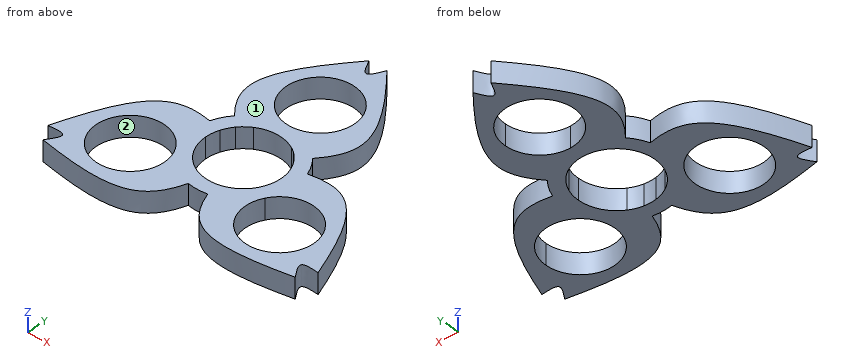
```python
from build123d import *

# Parameters (mm, degrees)
F0_R     = 9.95
F1_DEPTH = 6


with BuildPart() as f1:
    # F0 (on Top) → F1 (new body)
    with BuildSketch(Plane.XY):
        with BuildLine():
            ThreePointArc((5.5, 9.5262794416), (6.3093407999, 9.0106724872), (7.0706637066, 8.4264888743))
            ThreePointArc((7.0706637066, 8.4264888743), (7.8268557987, 7.7291867817), (8.5146077493, 6.9642985918))
            add(Edge.make_bspline(
                [(8.5146077493, 6.9642985918), (9.5301249028, 7.9008868503), (10.4822945034, 8.8485192108), (11.3460669028, 9.8115628642)],
                knots=[0.1806363612, 0.1806363612, 0.1806363612, 0.1806363612, 0.2520657546, 0.2520657546, 0.2520657546, 0.2520657546], degree=3))
            add(Edge.make_bspline(
                [(11.3460669028, 9.8115628642), (13.9736725709, 12.7411528396), (19.7429640918, 22.5358646022), (10.0301146668, 35.0297546933), (2.6054169788, 43.7370347171)],
                knots=[0.2520657546, 0.2520657546, 0.2520657546, 0.2520657546, 0.4693547987, 0.9448204936, 0.9448204936, 0.9448204936, 0.9448204936], degree=3))
            add(Edge.make_bspline(
                [(-2.6054169788, 43.7370347171), (-1.7369446525, 41.8435173586), (0, 38.0564826414), (1.7369446525, 41.8435173586), (2.6054169788, 43.7370347171)],
                knots=[0, 0, 0, 0, 0.5, 1, 1, 1, 1], degree=3))
            add(Edge.make_bspline(
                [(-11.3460669028, 9.8115628642), (-13.9736725709, 12.7411528396), (-19.7429640918, 22.5358646022), (-10.0301146668, 35.0297546933), (-2.6054169788, 43.7370347171)],
                knots=[0.2520657546, 0.2520657546, 0.2520657546, 0.2520657546, 0.4693547987, 0.9448204936, 0.9448204936, 0.9448204936, 0.9448204936], degree=3))
            add(Edge.make_bspline(
                [(-8.5146077493, 6.9642985918), (-9.5301249028, 7.9008868503), (-10.4822945034, 8.8485192108), (-11.3460669028, 9.8115628642)],
                knots=[0.1806363612, 0.1806363612, 0.1806363612, 0.1806363612, 0.2520657546, 0.2520657546, 0.2520657546, 0.2520657546], degree=3))
            ThreePointArc((-8.5146077493, 6.9642985918), (-7.1234292346, 8.381930323), (-5.5, 9.5262794416))
            ThreePointArc((-5.5, 9.5262794416), (0, 11), (5.5, 9.5262794416))
        make_face()
        with BuildLine():
            ThreePointArc((0, 15.05), (-7.0357124728, 32.0357124728), (9.95, 25))
            ThreePointArc((9.95, 25), (7.0357124728, 17.9642875272), (0, 15.05))
        make_face(mode=Mode.SUBTRACT)
        with BuildLine():
            add(Edge.make_bspline(
                [(8.5146077493, 6.9642985918), (9.5301249028, 7.9008868503), (10.4822945034, 8.8485192108), (11.3460669028, 9.8115628642)],
                knots=[0.1806363612, 0.1806363612, 0.1806363612, 0.1806363612, 0.2520657546, 0.2520657546, 0.2520657546, 0.2520657546], degree=3))
            ThreePointArc((8.5146077493, 6.9642985918), (9.5262794416, 5.5), (10.2885633747, 3.8917173182))
            add(Edge.make_bspline(
                [(10.2885633747, 3.8917173182), (11.6074311762, 4.3028868419), (12.9041896741, 4.6536737245), (14.1700961426, 4.9202007387)],
                knots=[0.1806363612, 0.1806363612, 0.1806363612, 0.1806363612, 0.2520657546, 0.2520657546, 0.2520657546, 0.2520657546], degree=3))
            ThreePointArc((14.1700961426, 4.9202007387), (12.9903810568, 7.5), (11.3460669028, 9.8115628642))
        make_face()
        with BuildLine():
            add(Edge.make_bspline(
                [(10.2885633747, 3.8917173182), (11.6074311762, 4.3028868419), (12.9041896741, 4.6536737245), (14.1700961426, 4.9202007387)],
                knots=[0.1806363612, 0.1806363612, 0.1806363612, 0.1806363612, 0.2520657546, 0.2520657546, 0.2520657546, 0.2520657546], degree=3))
            ThreePointArc((10.2885633747, 3.8917173182), (10.8206792098, 1.9781055177), (11, 0))
            ThreePointArc((11, 0), (9.5262794416, -5.5), (5.5, -9.5262794416))
            ThreePointArc((5.5, -9.5262794416), (3.6972499752, -10.3600358407), (1.7739556254, -10.85601591))
            add(Edge.make_bspline(
                [(1.7739556254, -10.85601591), (2.0773062734, -12.2037736923), (2.4218951707, -13.5021929353), (2.8240292398, -14.7317636029)],
                knots=[0.1806363612, 0.1806363612, 0.1806363612, 0.1806363612, 0.2520657546, 0.2520657546, 0.2520657546, 0.2520657546], degree=3))
            add(Edge.make_bspline(
                [(2.8240292398, -14.7317636029), (4.0473257472, -18.4721318504), (9.6451491958, -28.3658407506), (25.3216001194, -26.201211451), (36.5746746618, -24.1248746496)],
                knots=[0.2520657546, 0.2520657546, 0.2520657546, 0.2520657546, 0.4693547987, 0.9448204936, 0.9448204936, 0.9448204936, 0.9448204936], degree=3))
            add(Edge.make_bspline(
                [(36.5746746618, -24.1248746496), (35.3690766899, -22.4259968733), (32.9578807462, -19.0282413207), (37.1060213425, -19.4175204852), (39.1800916406, -19.6121600675)],
                knots=[0, 0, 0, 0, 0.5, 1, 1, 1, 1], degree=3))
            add(Edge.make_bspline(
                [(14.1700961426, 4.9202007387), (18.0209983181, 5.7309790107), (29.3881132876, 5.8299761484), (35.3517147861, -8.8285432423), (39.1800916406, -19.6121600675)],
                knots=[0.2520657546, 0.2520657546, 0.2520657546, 0.2520657546, 0.4693547987, 0.9448204936, 0.9448204936, 0.9448204936, 0.9448204936], degree=3))
        make_face()
        with BuildLine():
            ThreePointArc((13.033682327, -7.525), (24.2258845934, -2.8890380284), (31.6006350946, -12.5))
            ThreePointArc((31.6006350946, -12.5), (19.0753855958, -22.1109619716), (13.033682327, -7.525))
        make_face(mode=Mode.SUBTRACT)
        with BuildLine():
            ThreePointArc((-10.2885633747, 3.8917173182), (-9.5262794416, 5.5), (-8.5146077493, 6.9642985918))
            add(Edge.make_bspline(
                [(-8.5146077493, 6.9642985918), (-9.5301249028, 7.9008868503), (-10.4822945034, 8.8485192108), (-11.3460669028, 9.8115628642)],
                knots=[0.1806363612, 0.1806363612, 0.1806363612, 0.1806363612, 0.2520657546, 0.2520657546, 0.2520657546, 0.2520657546], degree=3))
            ThreePointArc((-11.3460669028, 9.8115628642), (-12.9903810568, 7.5), (-14.1700961426, 4.9202007387))
            add(Edge.make_bspline(
                [(-10.2885633747, 3.8917173182), (-11.6074311762, 4.3028868419), (-12.9041896741, 4.6536737245), (-14.1700961426, 4.9202007387)],
                knots=[0.1806363612, 0.1806363612, 0.1806363612, 0.1806363612, 0.2520657546, 0.2520657546, 0.2520657546, 0.2520657546], degree=3))
        make_face()
        with BuildLine():
            add(Edge.make_bspline(
                [(1.7739556254, -10.85601591), (2.0773062734, -12.2037736923), (2.4218951707, -13.5021929353), (2.8240292398, -14.7317636029)],
                knots=[0.1806363612, 0.1806363612, 0.1806363612, 0.1806363612, 0.2520657546, 0.2520657546, 0.2520657546, 0.2520657546], degree=3))
            ThreePointArc((1.7739556254, -10.85601591), (0, -11), (-1.7739556254, -10.85601591))
            add(Edge.make_bspline(
                [(-1.7739556254, -10.85601591), (-2.0773062734, -12.2037736923), (-2.4218951707, -13.5021929353), (-2.8240292398, -14.7317636029)],
                knots=[0.1806363612, 0.1806363612, 0.1806363612, 0.1806363612, 0.2520657546, 0.2520657546, 0.2520657546, 0.2520657546], degree=3))
            ThreePointArc((-2.8240292398, -14.7317636029), (0, -15), (2.8240292398, -14.7317636029))
        make_face()
        with BuildLine():
            ThreePointArc((-11, 0), (-10.8206792098, 1.9781055177), (-10.2885633747, 3.8917173182))
            add(Edge.make_bspline(
                [(-10.2885633747, 3.8917173182), (-11.6074311762, 4.3028868419), (-12.9041896741, 4.6536737245), (-14.1700961426, 4.9202007387)],
                knots=[0.1806363612, 0.1806363612, 0.1806363612, 0.1806363612, 0.2520657546, 0.2520657546, 0.2520657546, 0.2520657546], degree=3))
            add(Edge.make_bspline(
                [(-14.1700961426, 4.9202007387), (-18.0209983181, 5.7309790107), (-29.3881132876, 5.8299761484), (-35.3517147861, -8.8285432423), (-39.1800916406, -19.6121600675)],
                knots=[0.2520657546, 0.2520657546, 0.2520657546, 0.2520657546, 0.4693547987, 0.9448204936, 0.9448204936, 0.9448204936, 0.9448204936], degree=3))
            add(Edge.make_bspline(
                [(-39.1800916406, -19.6121600675), (-37.1060213425, -19.4175204852), (-32.9578807462, -19.0282413207), (-35.3690766899, -22.4259968733), (-36.5746746618, -24.1248746496)],
                knots=[0, 0, 0, 0, 0.5, 1, 1, 1, 1], degree=3))
            add(Edge.make_bspline(
                [(-2.8240292398, -14.7317636029), (-4.0473257472, -18.4721318504), (-9.6451491958, -28.3658407506), (-25.3216001194, -26.201211451), (-36.5746746618, -24.1248746496)],
                knots=[0.2520657546, 0.2520657546, 0.2520657546, 0.2520657546, 0.4693547987, 0.9448204936, 0.9448204936, 0.9448204936, 0.9448204936], degree=3))
            add(Edge.make_bspline(
                [(-1.7739556254, -10.85601591), (-2.0773062734, -12.2037736923), (-2.4218951707, -13.5021929353), (-2.8240292398, -14.7317636029)],
                knots=[0.1806363612, 0.1806363612, 0.1806363612, 0.1806363612, 0.2520657546, 0.2520657546, 0.2520657546, 0.2520657546], degree=3))
            ThreePointArc((-1.7739556254, -10.85601591), (-3.6972499752, -10.3600358407), (-5.5, -9.5262794416))
            ThreePointArc((-5.5, -9.5262794416), (-9.5262794416, -5.5), (-11, 0))
        make_face()
        with Locations((-21.6506350946, -12.5)):
            Circle(F0_R, mode=Mode.SUBTRACT)
    extrude(amount=F1_DEPTH)


solid = f1.part
```
Geometry check sheet. Reference: the model listing, model coordinates, mm. Face numbers are marked on the shaded views. Coordinates: 2 decimals unless noted, no trailing zeros. Answer in a Markdown table with one row per item. Add a question column.
1. Gauge pin test, flat ends, axial feed: pin 1 Ø2 at (x, z) = (28, 1) entering from +Y; pin 2 Ø1 at (y, z) = (-12.5, 4) entering from -X; pin 3 Ø2 at (y, z) = (11, 3.5) entering from -X. Record the tip position at first contact, or that the pin passes through.
2. Draft check along Y on the marked faces 1 and 2. Enter one of: +Y half, -Y half, draft (parallel to the pull), parting line (faces both ways), or undercut.
3. Section check A-A (x = -13). Give the number of separate pieces and of enclosed holes in the cut face, plus the area to 3 significant figures.
4. Material ranges on L1, parallel to Y at x = 0, z = 3.3; L2, parallel to Y at x = -6.5, z = 4.5; L3, parallel to X at y = -20.5, z = 5.5, recorded low to high. Write a range as [from, to].
Data:
| question | item | result |
|---|---|---|
| 1 | pin 1 | stops at y = 2.86 |
| 1 | pin 2 | stops at x = -36.72 |
| 1 | pin 3 | stops at x = -13.13 |
| 2 | face 1 | draft |
| 2 | face 2 | undercut |
| 3 | separate pieces | 3 |
| 3 | enclosed holes | 0 |
| 3 | area | 247 mm² |
| 4 | L1 | y = [-15, -11], [11, 15.05], [34.95, 39.95] |
| 4 | L2 | y = [-21.65, -8.87], [8.87, 17.47], [32.53, 39.06] |
| 4 | L3 | x = [-34.52, -27.57], [-15.73, -5.59], [5.59, 15.73], [27.57, 34.52] |
